Read the model definition and answer for the solid it produces. Units are mm, in the model's axes. Face numbers are marked on the shaded views. Coordinates: 2 decimals unless noted, no trailing zeros. Order: outer loops, then holes, each group sorted by start corner. A loop starts at its lowest first (then second) coordinate and runs counter-clockwise, first axis right, second up. Notation, with made-up numbers: M 25.25,84 L 30.25,84 A36 cw 30.25,118 Z; hole C -8,-30.5 d4. An arc over 180 degrees is marked long. Use a Markdown table: item, result. Add a question column.
1) The mould has two halves that part along Y. Classify the marked faces 1, 2 and 3: released by +Y, released by -Y, zero draft, split by the parting line, or undercut.
2) Find section B-B on y = 0. Write down the section's boundary in (x, z) (3 decimals).
3) Find section C-C on z = 21.5. Write down the section's boundary in (x, y).
4) Find the intervals of material crossed by probe 1 along Z at (x, y) = (12, -2); probe 2 along Y at (x, z) = (0, -2.5) (3 decimals); probe 3 along Y at (x, z) = (0, 25.5), in increasing order. Write a range as [from, to].
5) Find section A-A on x = 7.5. Write down the section's boundary in (y, z).
6) Each of these flat-tipped pins is pushed along its axis until it touches: pin 1 Ø3 at (y, z) = (-1, -1) entering from +X; pin 2 Ø1.5 at (y, z) = (-10.5, -18.5) entering from +X; pin 3 Ø6 at (y, z) = (8.5, -14) entering from +X; pin 4 Ø8 at (y, z) = (-9.5, 5.5) entering from -X. Where does it stop, or does it pass through?
from build123d import *

# Parameters (mm, degrees)
EXTRUDE1_DEPTH       = 36.143
EXTRUDE1_DEPTH_BACK  = 36.143
SKETCH1_R            = 16.7
STROKE_START         = -15.2
SKETCH2_R            = 15.875
STROKE_CHAMBER_DEPTH = 30.4
ROD_HOLE_REACH       = 78.046
SKETCH3_R            = 5.6


with BuildPart() as part:
    # Sketch1 → Extrude1 (new, two sides: drawn at the far end of the back side and taken through both)
    with BuildSketch(Plane.XY.offset(-EXTRUDE1_DEPTH_BACK)):
        Circle(SKETCH1_R)
    extrude(amount=EXTRUDE1_DEPTH + EXTRUDE1_DEPTH_BACK)

    # Sketch2 → STROKE CHAMBER (cut)
    with BuildSketch(Plane.XY.offset(STROKE_START)):
        Circle(SKETCH2_R)
    extrude(amount=STROKE_CHAMBER_DEPTH, mode=Mode.SUBTRACT)

    # Sketch3 → ROD HOLE (cut, up to next)
    with BuildSketch(Plane.XY.offset(36.143), mode=Mode.PRIVATE) as rod_hole_sk1:
        Circle(SKETCH3_R)
    rod_hole_tool1 = extrude(rod_hole_sk1.sketch, amount=-ROD_HOLE_REACH, mode=Mode.PRIVATE) & part.part
    add(rod_hole_tool1.solids().sort_by_distance((0, 0, 36.143))[0], mode=Mode.SUBTRACT)


solid = part.part
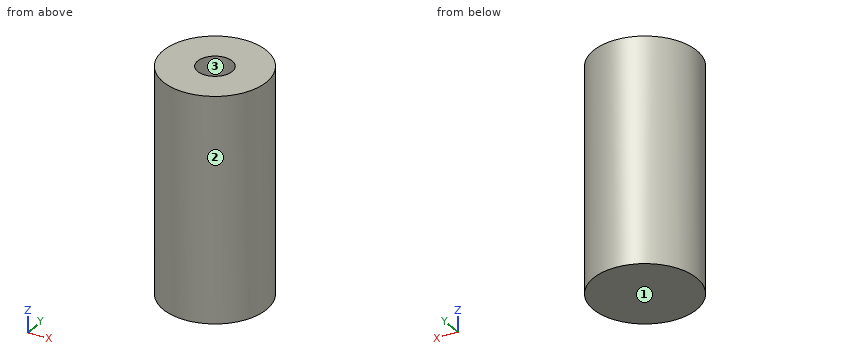
Check result:
| question | item | result |
|---|---|---|
| 1 | face 1 | zero draft |
| 1 | face 2 | split by the parting line |
| 1 | face 3 | undercut |
| 2 | outline | M -16.7,-36.143 L 16.7,-36.143 L 16.7,36.143 L 5.6,36.143 L 5.6,15.2 L 15.875,15.2 L 15.875,-15.2 L -15.875,-15.2 L -15.875,15.2 L -5.6,15.2 L -5.6,36.143 L -16.7,36.143 Z |
| 3 | outline | C 0,0 d33.4; hole C 0,0 d11.2 |
| 4 | probe 1 | z = [-36.14, -15.2], [15.2, 36.14] |
| 4 | probe 2 | y = [-16.7, -15.875], [15.875, 16.7] |
| 4 | probe 3 | y = [-16.7, -5.6], [5.6, 16.7] |
| 5 | outline | M -14.92,-36.14 L 14.92,-36.14 L 14.92,36.14 L -14.92,36.14 Z; hole M -13.99,-15.2 L 13.99,-15.2 L 13.99,15.2 L -13.99,15.2 Z |
| 6 | pin 1 | stops at x = 16.7 |
| 6 | pin 2 | stops at x = 13.56 |
| 6 | pin 3 | stops at x = 15.77 |
| 6 | pin 4 | stops at x = -15.77 |
